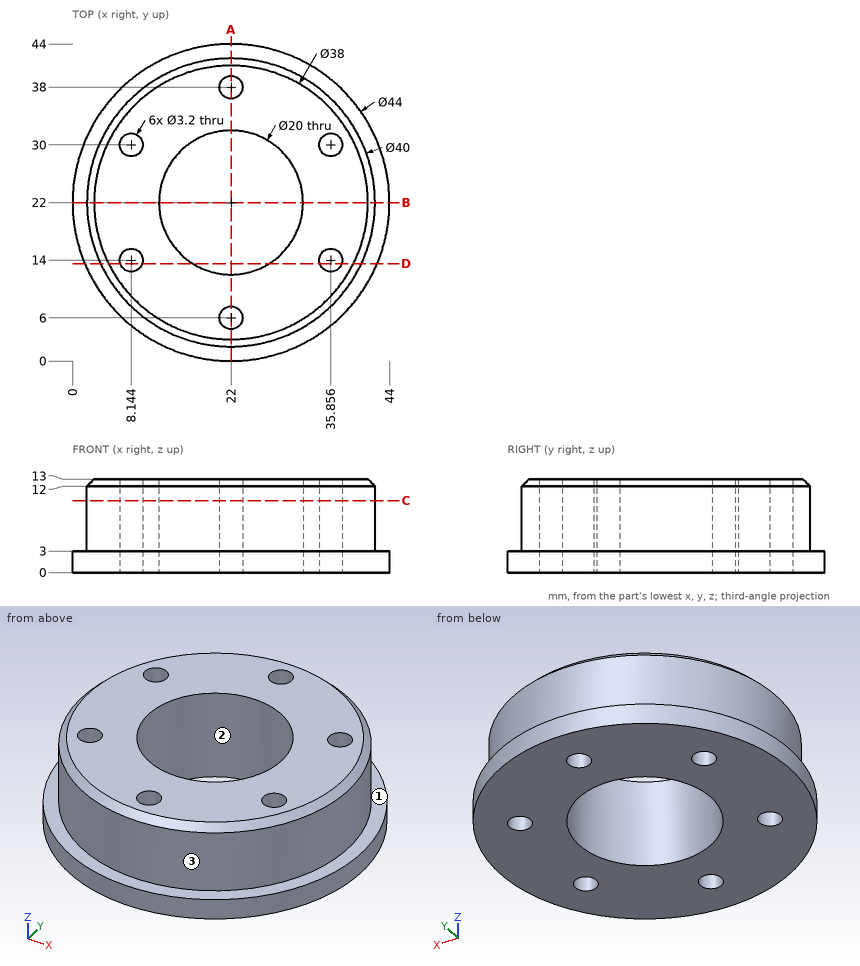
Input: dimensioned drawing with shaded views. Units: mm. Origin: part minimum x, y, z. Coordinates: 2 decimals unless noted, no trailing zeros. Order: outer loops, then holes, each group sorted by start corner. A loop starts at its lowest first (then second) coordinate and runs counter-clockwise, first axis right, second up.
1. Cut plane B-B, the plane y = 22. Return loops of the section in (x, z), plus the area to 3 significant figures.
Checked values:
outline: (0, 0) - (12, 0) - (12, 13) - (3, 13) - (2, 12) - (2, 3) - (0, 3) - close; (32, 0) - (44, 0) - (44, 3) - (42, 3) - (42, 12) - (41, 13) - (32, 13) - close
area: 271 mm2
2. Contact query for flat-ended pins moving along their axis: P1, Ø1.5, axis at x = 20.5, z = 8, coming from the +Y side; P2, Ø5, axis at x = 13.5, z = 5, coming from the +Y side; P3, Ø1.5, axis at y = 27, z = 5.5, coming from the +X side. Output: stop coordinate, or through.
Checked values:
P1: stops at y = 41.99
P2: stops at y = 42.86
P3: stops at x = 41.54
3. Cut plane A-A, the plane x = 22. Return loops of the section in (y, z).
Checked values:
outline: (0, 0) - (4.4, 0) - (4.4, 13) - (3, 13) - (2, 12) - (2, 3) - (0, 3) - close; (7.6, 0) - (12, 0) - (12, 13) - (7.6, 13) - close; (32, 0) - (36.4, 0) - (36.4, 13) - (32, 13) - close; (39.6, 0) - (44, 0) - (44, 3) - (42, 3) - (42, 12) - (41, 13) - (39.6, 13) - close
4. Cut plane D-D, the plane y = 13.5. Count the separate pieces of the cut face and the enclosed holes in it, plus the area to 3 significant figures.
Checked values:
separate pieces: 4
enclosed holes: 0
area: 267 mm2
5. Ray query, line 1 along Y through (x, z) = (22, 3.5); line 2 along X through (y, z) = (14, 9.5) (1 decimal); line 3 along X through (y, z) = (22, 10). Return the intervals inside material, ascending.
Checked values:
line 1: y = 2 to 4.4, 7.6 to 12, 32 to 36.4, 39.6 to 42
line 2: x = 3.7 to 6.5, 9.7 to 16, 28 to 34.3, 37.5 to 40.3
line 3: x = 2 to 12, 32 to 42
6. Draft query along Y for the marked faces 1, 2 and 3. Return one class per face: +Y half, -Y half, draft (parallel to the pull), parting line (faces both ways), or undercut.
Checked values:
face 1: draft
face 2: undercut
face 3: parting line
7. Cut plane C-C, the plane z = 10. Return loops of the section in (x, y).
Checked values:
outline: circle Ø40 at (22, 22); hole circle Ø3.2 at (8.14, 14); hole circle Ø3.2 at (8.14, 30); hole circle Ø20 at (22, 22); hole circle Ø3.2 at (22, 6); hole circle Ø3.2 at (22, 38); hole circle Ø3.2 at (35.86, 14); hole circle Ø3.2 at (35.86, 30)
